Here's how the part is built. I have some questions about the finished solid (model axes, mm). Face numbers are marked on the shaded views. A direction names the side the tool comes from. Coordinates: 2 decimals unless noted, no trailing zeros. Order: outer loops, then holes, each group sorted by start corner. A loop starts at its lowest first (then second) coordinate and runs counter-clockwise, first axis right, second up. Notation, with made-up numbers: (11.25, 21) - (50.25, 21) arc R32 ccw to (50.25, 51) - close; hole circle Ø6 at (-4, 26). An arc over 180 degrees is marked (long way). Answer in a Markdown table with one row per item. Add a question column.
Item 1: Will these pins go through, and if not, where does the flat tip stop? pin 1 Ø4 at (x, y) = (-27.5, 56) entering from -Z; pin 2 Ø8 at (x, y) = (-21, 68) entering from +Z; pin 3 Ø1.5 at (x, z) = (-48, 21) entering from +Y; pin 4 Ø1.5 at (x, z) = (-41.5, 35.5) entering from +Y.
Item 2: If I drill on line 1 along X through (y, z) = (36, 40); line 2 along Z through (x, y) = (-4, 30.5); line 3 along Y through (x, z) = (-33, 24), over which ranges is the centre line in solid material (lowest first)? Write a range as from..to.
Item 3: I want a section at B-B (y = 34.5). Please give me the cut outline in (x, z).
Item 4: I want a section at D-D (x = -14.5). Please give me the cut outline in (y, z).
Item 5: On a 3-axis mill with a long thin cutter (end or side, diameter ignored), from which of +Z, -Z, +X, -X, +Y, -Y can I reach the whole of each face in a straight line? I mean the marked faces 4 and 5. Say none if no direction works.
Item 6: I want a section at A-A (x = -43.5). Please give me the cut outline in (y, z).
Item 7: I want a section at C-C (z = 3.5). Please give me the cut outline in (x, y), plus the area to 3 significant figures.
Item 8: Thinking about a two-plate mould opening in X: for the marked faces 1, 2 and 3, which applies, +X half, -X half, draft (parallel to the pull), parting line (faces both ways), or undercut?
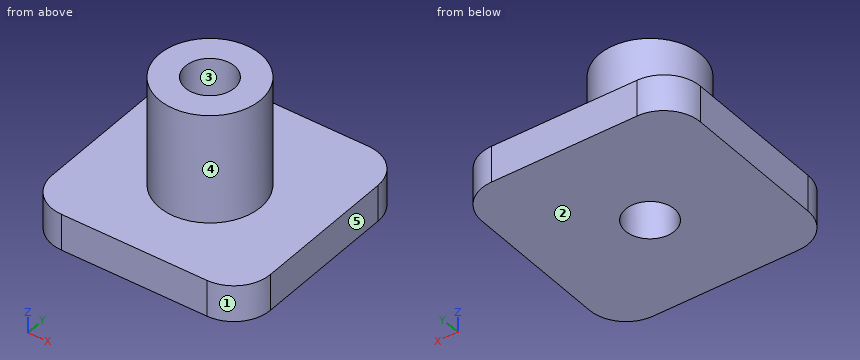
```python
from build123d import *

# Parameters (mm, degrees)
F0_R     = 17.679544
F1_DEPTH = 12.7
F0_R_2   = 8.543995
F2_DEPTH = 50.8


with BuildPart() as f1:
    # F0 (on Top) → F1 (new body)
    with BuildSketch(Plane.XY):
        with BuildLine():
            Line((-63.5, 0), (-12.7, 0))
            ThreePointArc((-12.7, 0), (-3.719744, 3.719744), (0, 12.7))
            Line((0, 12.7), (0, 63.5))
            ThreePointArc((0, 63.5), (-3.719744, 72.480256), (-12.7, 76.2))
            Line((-12.7, 76.2), (-63.5, 76.2))
            ThreePointArc((-63.5, 76.2), (-72.480256, 72.480256), (-76.2, 63.5))
            Line((-76.2, 63.5), (-76.2, 12.7))
            ThreePointArc((-76.2, 12.7), (-72.480256, 3.719744), (-63.5, 0))
        make_face()
        with Locations((-38.140807, 35.769224)):
            Circle(F0_R, mode=Mode.SUBTRACT)
    extrude(amount=F1_DEPTH)

    # F0 (on Top) → F2 (join)
    with BuildSketch(Plane.XY):
        with Locations((-38.140807, 35.769224)):
            Circle(F0_R)
        with Locations((-38.140807, 35.769224)):
            Circle(F0_R_2, mode=Mode.SUBTRACT)
    extrude(amount=F2_DEPTH)


solid = f1.part
```
Values follow:
| question | item | result |
|---|---|---|
| 1 | pin 1 | stops at z = 0 |
| 1 | pin 2 | stops at z = 12.7 |
| 1 | pin 3 | stops at y = 50.92 |
| 1 | pin 4 | stops at y = 53.26 |
| 2 | line 1 | x = -55.82..-46.68, -29.6..-20.46 |
| 2 | line 2 | z = 0..12.7 |
| 2 | line 3 | y = 18.85..28.94, 42.59..52.68 |
| 3 | outline | (-76.2, 0) - (-46.59, 0) - (-46.59, 50.8) - (-55.77, 50.8) - (-55.77, 12.7) - (-76.2, 12.7) - close; (-29.69, 0) - (0, 0) - (0, 12.7) - (-20.51, 12.7) - (-20.51, 50.8) - (-29.69, 50.8) - close |
| 4 | outline | (0, 0) - (76.2, 0) - (76.2, 12.7) - (0, 12.7) - close |
| 5 | face 4 | +Z |
| 5 | face 5 | +Z, -Z, +X, +Y, -Y |
| 6 | outline | (0, 0) - (29.11, 0) - (29.11, 50.8) - (18.92, 50.8) - (18.92, 12.7) - (0, 12.7) - close; (42.42, 0) - (76.2, 0) - (76.2, 12.7) - (52.62, 12.7) - (52.62, 50.8) - (42.42, 50.8) - close |
| 7 | outline | (-76.2, 12.7) arc R12.7 ccw to (-63.5, 0) - (-12.7, 0) arc R12.7 ccw to (0, 12.7) - (0, 63.5) arc R12.7 ccw to (-12.7, 76.2) - (-63.5, 76.2) arc R12.7 ccw to (-76.2, 63.5) - close; hole circle Ø17.09 at (-38.14, 35.77) |
| 7 | area | 5,440 mm^2 |
| 8 | face 1 | +X half |
| 8 | face 2 | draft |
| 8 | face 3 | undercut |
